Model file for the job. Use its own axes, mm. Face numbers are marked on the shaded views. Round coordinates to 2 decimals unless told otherwise and drop trailing zeros. Order: outer loops, then holes, each group sorted by start corner. A loop starts at its lowest first (then second) coordinate and runs counter-clockwise, first axis right, second up. Notation, with made-up numbers: (34, 46) - (68, 46) arc R31 cw to (68, 72) - close; hole circle Ø11 at (55, -19.75). An arc over 180 degrees is marked (long way). Put each result on its own line as item: value. Start each with the question number.
Item 1: Saw through at A-A on x = -1.75. List the corners of the cut face in (y, z) (3 decimals), plus the area to 3 significant figures.
Item 2: Probe probe 1 along Y at (x, z) = (-4.5, 17.5) (3 decimals); probe 2 along Z at (x, y) = (-2, -2.5); probe 3 along Y at (x, z) = (-13.6, -21). List the from-to ranges inside material, lowest first.
Item 3: Pin check, flat tip, straight feed: pin 1 Ø2 at (y, z) = (0, -21) entering from +X. Stop position of the tip, or through.
Item 4: Saw through at C-C on y = 4.5. List the corners of the cut face in (x, z), plus the area to 3 significant figures.
Item 5: Saw through at D-D on z = 10.5. List the corners of the cut face in (x, y) (3 decimals).
Item 6: Saw through at B-B on z = -21. List the corners of the cut face in (x, y).
Item 7: Mould opens along Z. For the marked faces 1, 2 and 3 say: pulls with the +Z half, pulls with the -Z half, needs draft (parallel to the pull), parting line crosses it, or undercut.
Autodesk Inventor part; units mm, degrees
ref_plane "YZ Plane" through (0, 0, 0) normal (1, 0, 0) x (0, 1, 0)
ref_plane "XZ Plane" through (0, 0, 0) normal (0, 1, 0) x (-1, 0, 0)
ref_plane "XY Plane" through (0, 0, 0) normal (0, 0, 1) x (1, 0, 0)
sketch "スケッチ2" plane through (0, -6.5, -24) normal (-1, 0, 0) x (0, 0, 1)
  arc A0 (2.5, 15.5) -> (0, 13) centre (2.5, 13) ccw
  line L0 (0, 0) -> (0, 13)
  arc A1 (0, 0) -> (2.5, -2.5) centre (2.5, 0) ccw
  line L1 (45.5, -2.5) -> (2.5, -2.5)
  arc A2 (45.5, -2.5) -> (48, 0) centre (45.5, 0) ccw
  line L2 (48, 13) -> (48, 0)
  arc A3 (48, 13) -> (45.5, 15.5) centre (45.5, 13) ccw
  line L3 (2.5, 15.5) -> (45.5, 15.5)
  point P0 (24, 6.5)
extrude "押し出し2" add sketch "スケッチ2" along normal blind 15
sketch "スケッチ1" plane through (-15, -6.5, -24) normal (-1, 0, 0) x (0, 0, 1)
  line L0 (24, 6.5) -> (24, -15.1868) construction
  circle A0 centre (45, 6.5) radius 0.8
  circle A1 centre (3, 6.5) radius 0.8
  line L1 (45, 6.5) -> (24, 6.5) construction
  dimension "d0" = 1.6
  dimension "d1" = 42
extrude "押し出し1" cut sketch "スケッチ1" against normal blind 5.5
sketch "スケッチ3" plane through (0, -6.5, -24) normal (-1, 0, 0) x (0, 0, -1)
  line L0 (-33.2, -7.925) -> (-43, -7.925)
  line L1 (-43, -7.925) -> (-43, 0.425)
  line L2 (-43, 0.425) -> (-30.55, 0.425)
  line L3 (-30.55, 0.425) -> (-30.55, -3.425)
  line L4 (-30.55, -3.425) -> (-33.2, -3.425)
  line L5 (-33.2, -3.425) -> (-33.2, -7.925)
  line L6 (-43, -13.425) -> (-43, -8.925)
  line L7 (-43, -8.925) -> (-33.2, -8.925)
  line L8 (-33.2, -8.925) -> (-33.2, -13.425)
  line L9 (-33.2, -13.425) -> (-43, -13.425)
  point P0 (-24, -6.5)
extrude "押し出し3" cut sketch "スケッチ3" along normal blind 5
fillet "フィレット1" radius 1 8 edges at (0, 8.2678, -23.2678) (0, 0, -24) (0, -8.2678, -23.2678) (0, -9, 0) (0, -8.2678, 23.2678) (0, 0, 24) (0, 8.2678, 23.2678) (0, 9, 0)
sketch "スケッチ4" plane through (-15, -6.5, -24) normal (0, 0, -1) x (-1, 0, 0)
  line L0 (-11.15, 2.5) -> (-8.15, 2.5)
  line L1 (-8.15, 2.5) -> (-8.15, 10.5)
  line L2 (-8.15, 10.5) -> (-11.15, 10.5)
  line L3 (-11.15, 10.5) -> (-11.15, 2.5)
  line L4 (-15, 6.5) -> (-11.15, 6.5) construction
  dimension "d9" = 8
  dimension "d10" = 3
  dimension "d11" = 3.85
extrude "押し出し4" cut sketch "スケッチ4" against normal blind 5
properties part number "U2D2" material "ABS プラスチック"
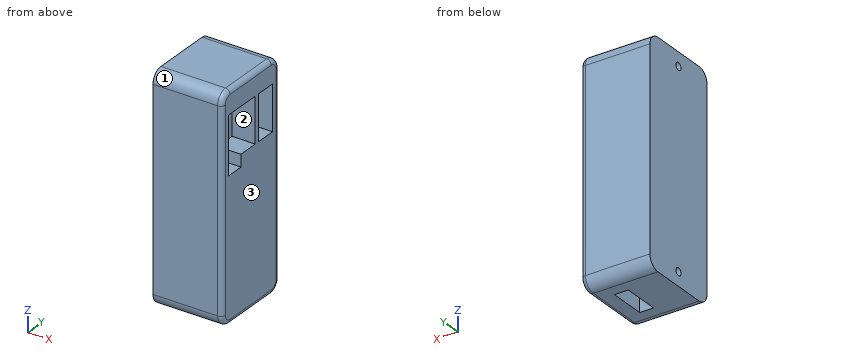
Results found:
1. outline: (-9, -21.5) arc R2.5 ccw to (-6.5, -24) - (6.5, -24) arc R2.5 ccw to (9, -21.5) - (9, 21.5) arc R2.5 ccw to (6.5, 24) - (-6.5, 24) arc R2.5 ccw to (-9, 21.5) - close; hole (-6.925, 6.55) - (-3.075, 6.55) - (-3.075, 9.2) - (1.425, 9.2) - (1.425, 19) - (-6.925, 19) - close; hole (2.425, 9.2) - (6.925, 9.2) - (6.925, 19) - (2.425, 19) - close
1. area: 723 mm²
2. probe 1: y = -9 to -6.925, 1.425 to 2.425, 6.925 to 9
2. probe 2: z = -24 to 9.2, 19 to 24
2. probe 3: y = -9 to -0.8, 0.8 to 9
3. pin 1: stops at x = 0
4. outline: (-15, -24) - (-1, -24) arc R1 ccw to (0, -23) - (0, 9.2) - (-5, 9.2) - (-5, 19) - (0, 19) - (0, 23) arc R1 ccw to (-1, 24) - (-15, 24) - close
4. area: 671 mm²
5. outline: (-15, -9) - (-1, -9) arc R1 ccw to (0, -8) - (0, -6.925) - (-5, -6.925) - (-5, 1.425) - (0, 1.425) - (0, 2.425) - (-5, 2.425) - (-5, 6.925) - (0, 6.925) - (0, 8) arc R1 ccw to (-1, 9) - (-15, 9) - close
6. outline: (-15, -9) - (-1, -9) arc R1 ccw to (0, -8) - (0, 8) arc R1 ccw to (-1, 9) - (-15, 9) - (-15, 0.8) - (-9.5, 0.8) - (-9.5, -0.8) - (-15, -0.8) - close; hole (-6.85, -4) - (-3.85, -4) - (-3.85, 4) - (-6.85, 4) - close
7. face 1: pulls with the +Z half
7. face 2: undercut
7. face 3: needs draft
